CAD build for the part. Positions are in the model's coordinates, mm. Face numbers are marked on the shaded views. A direction names the side the tool comes from. Give positions to 0.01 mm unless a question says otherwise; leave off trailing zeros. Order: outer loops, then holes, each group sorted by start corner. A loop starts at its lowest first (then second) coordinate and runs counter-clockwise, first axis right, second up.
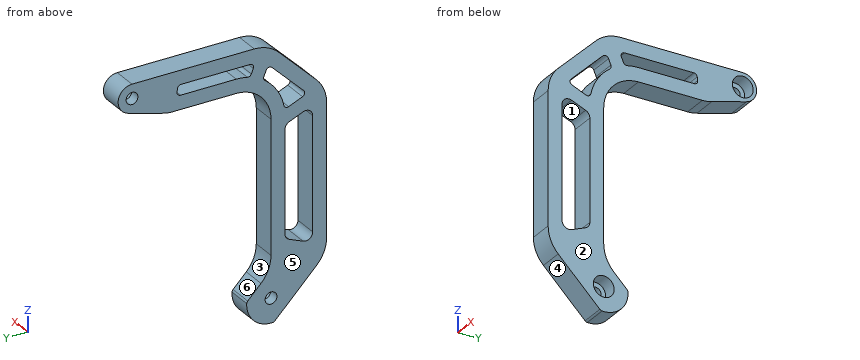
Autodesk Inventor part; units mm, degrees
ref_plane "YZ Plane" through (0, 0, 0) normal (1, 0, 0) x (0, 1, 0)
ref_plane "XZ Plane" through (0, 0, 0) normal (0, 1, 0) x (-1, 0, 0)
ref_plane "XY Plane" through (0, 0, 0) normal (0, 0, 1) x (1, 0, 0)
sketch "SwingArm A" plane through (0, 0, 0) normal (0, 0, 1) x (1, 0, 0)
  line L0 (-13.1129, 5.4447) -> (-1.1226, -6.6888)
  arc A0 (6.9887, 0.3969) -> (6.7016, 1.0431) centre (5.9903, 0.3402) ccw
  arc A1 (-1.1226, -6.6888) -> (-0.4798, -6.9835) centre (-0.4113, -5.9859) ccw
  line L1 (40, 71) -> (4.8211, 71)
  line L2 (28.3926, 60) -> (0, 60) construction
  line L3 (-2.2079, 68.1129) -> (-13.029, 57.4195)
  line L4 (-16, 50.3066) -> (-16, 12.4737)
  line L5 (0, 60) -> (0, 11.9322) construction
  line L6 (2.8871, 4.9032) -> (6.7016, 1.0431)
  circle A2 centre (0, 0) radius 1.7
  circle A3 centre (40, 67) radius 1.7
  line L7 (40, 67) -> (-8, 67) construction
  line L8 (-8, 67) -> (-8, 8.0955) construction
  line L9 (-8, 8.0955) -> (0, 0) construction
  line L10 (41.0716, 63.1462) -> (31.0716, 60.3655)
  arc A4 (28.3926, 60) -> (31.0716, 60.3655) centre (28.3926, 70) ccw
  circle A5 centre (40, 67) radius 4 construction
  arc A6 (41.0716, 63.1462) -> (40, 71) centre (40, 67) ccw
  circle A7 centre (0, 0) radius 5.5 construction
  arc A8 (10, 60) -> (0, 50) centre (10, 50) ccw
  arc A9 (0, 11.9322) -> (2.8871, 4.9032) centre (10, 11.9322) ccw
  arc A10 (-16, 12.4737) -> (-13.1129, 5.4447) centre (-6, 12.4737) ccw
  arc A11 (-13.029, 57.4195) -> (-16, 50.3066) centre (-6, 50.3066) ccw
  arc A12 (4.8211, 71) -> (-2.2079, 68.1129) centre (4.8211, 61) ccw
  line L11 (-9.2401, 13.305) -> (-5.2401, 14.948)
  line L12 (-4, 16.798) -> (-4, 45.9717)
  line L13 (-5.2292, 47.8172) -> (-9.2292, 49.488)
  line L14 (-12, 47.6425) -> (-12, 15.155)
  arc A13 (-4, 45.9717) -> (-5.2292, 47.8172) centre (-6, 45.9717) ccw
  arc A14 (-9.2292, 49.488) -> (-12, 47.6425) centre (-10, 47.6425) ccw
  arc A15 (-5.2401, 14.948) -> (-4, 16.798) centre (-6, 16.798) ccw
  arc A16 (-12, 15.155) -> (-9.2401, 13.305) centre (-10, 15.155) ccw
  line L15 (28.3926, 60) -> (10, 60)
  line L16 (0, 50) -> (0, 11.9322)
  line L17 (1.3855, 64.1003) -> (2.0531, 62.4749)
  line L18 (-5.0798, 52.0897) -> (-9.0729, 53.7576)
  line L19 (-0.2424, 64.4316) -> (-9.3904, 55.3916)
  arc A17 (1.7195, 61.2887) -> (2.0531, 62.4749) centre (1.1281, 62.095) ccw
  arc A18 (1.3855, 64.1003) -> (-0.2424, 64.4316) centre (0.4605, 63.7204) ccw
  arc A19 (-5.0798, 52.0897) -> (-3.7148, 52.8116) centre (-4.6944, 53.0125) ccw
  arc A20 (-9.3904, 55.3916) -> (-9.0729, 53.7576) centre (-8.6875, 54.6803) ccw
  line L20 (-15.2274, 54.1608) -> (0, 47.8005) construction
  arc A21 (-0.4798, -6.9835) -> (6.9887, 0.3969) centre (0, 0) ccw
  arc A22 (1.7195, 61.2887) -> (-3.7148, 52.8116) centre (10, 50) ccw
  line L21 (0.0419, 2.0916) -> (2.8931, -0.7936) construction
  arc A23 (0.7592, -2.9023) -> (2.8931, -0.7936) centre (0, 0) ccw construction
  line L22 (0.7592, -2.9023) -> (-10.2677, 8.2563) construction
  arc A24 (-12, 12.4737) -> (-10.2677, 8.2563) centre (-6, 12.4737) ccw construction
  line L23 (-12, 12.4737) -> (-12, 50.3066) construction
  arc A25 (-10.2174, 54.5744) -> (-12, 50.3066) centre (-6, 50.3066) ccw construction
  line L24 (-10.2174, 54.5744) -> (0.6037, 65.2677) construction
  arc A26 (4.8211, 67) -> (0.6037, 65.2677) centre (4.8211, 61) ccw construction
  line L25 (4.8211, 67) -> (40, 67) construction
  line L26 (40, 67) -> (30, 64.2193) construction
  arc A27 (28.3926, 64) -> (30, 64.2193) centre (28.3926, 70) ccw construction
  line L27 (28.3926, 64) -> (10, 64) construction
  arc A28 (10, 64) -> (-4, 50) centre (10, 50) ccw construction
  line L28 (-4, 50) -> (-4, 11.9322) construction
  arc A29 (-4, 11.9322) -> (0.0419, 2.0916) centre (10, 11.9322) ccw construction
  line L29 (-15.2501, 8.6743) -> (0, 14.9381) construction
  line L30 (1.0217, 70.2501) -> (5.6423, 59.0006) construction
  line L31 (29.7445, 60.0918) -> (28.2561, 71) construction
  line L32 (5.6582, 64.2257) -> (5.0855, 65.6201)
  line L33 (26.9014, 66.1352) -> (27.0378, 65.1352)
  line L34 (25.9106, 67) -> (6.0106, 67)
  line L35 (26.047, 64) -> (10, 64)
  arc A30 (10, 64) -> (6.811, 63.632) centre (10, 50) ccw
  arc A31 (5.6582, 64.2257) -> (6.811, 63.632) centre (6.5833, 64.6057) ccw
  arc A32 (6.0106, 67) -> (5.0855, 65.6201) centre (6.0106, 66) ccw
  arc A33 (26.9014, 66.1352) -> (25.9106, 67) centre (25.9106, 66) ccw
  arc A34 (26.047, 64) -> (27.0378, 65.1352) centre (26.047, 65) ccw
  point P0 (-12, 31.3902)
  point P1 (-16, 31.3902)
  dimension "d0" = 3.4
  dimension "d1" = 3.4
  dimension "d2" = 7
  dimension "d3" = 4
  dimension "d6" = 10
  dimension "d7" = 16
  dimension "d8" = 67
  dimension "d9" = 10
  dimension "d10" = 10
  dimension "d11" = 10
  dimension "d12" = 10
  dimension "d13" = 10
  dimension "d14" = 40
  dimension "d15" = 134.66
  dimension "d16" = 2
  dimension "d17" = 2
  dimension "d18" = 1
  dimension "d20" = 4
  dimension "d24" = 10
  dimension "d25" = 50
  dimension "d32" = 7
  dimension "d33" = 11
  dimension "d34" = 1
  dimension "d35" = 4
  dimension "d37" = 2
  dimension "d38" = 4
  dimension "d39" = 1
  dimension "d41" = 2
  dimension "d42" = 1
  dimension "d43" = 1
sketch "Skizze1" plane through (0, 0, 0) normal (1, 0, 0) x (0, 1, 0)
  circle A0 centre (40, 67) radius 3
  circle A1 centre (0, 0) radius 3
  line L0 (-13.1129, 5.4447) -> (-1.1226, -6.6888)
  arc A2 (6.9887, 0.3969) -> (6.7016, 1.0431) centre (5.9903, 0.3402) ccw
  arc A3 (-1.1226, -6.6888) -> (-0.4798, -6.9835) centre (-0.4113, -5.9859) ccw
  line L1 (40, 71) -> (4.8211, 71)
  line L2 (28.3926, 60) -> (0, 60) construction
  line L3 (-2.2079, 68.1129) -> (-13.029, 57.4195)
  line L4 (-16, 50.3066) -> (-16, 12.4737)
  line L5 (0, 60) -> (0, 11.9322) construction
  line L6 (2.8871, 4.9032) -> (6.7016, 1.0431)
  circle A4 centre (0, 0) radius 1.7
  circle A5 centre (40, 67) radius 1.7
  line L7 (40, 67) -> (-8, 67) construction
  line L8 (-8, 67) -> (-8, 8.0955) construction
  line L9 (-8, 8.0955) -> (0, 0) construction
  line L10 (41.0716, 63.1462) -> (31.0716, 60.3655)
  arc A6 (28.3926, 60) -> (31.0716, 60.3655) centre (28.3926, 70) ccw
  circle A7 centre (40, 67) radius 4 construction
  arc A8 (41.0716, 63.1462) -> (40, 71) centre (40, 67) ccw
  circle A9 centre (0, 0) radius 5.5 construction
  arc A10 (10, 60) -> (0, 50) centre (10, 50) ccw
  arc A11 (0, 11.9322) -> (2.8871, 4.9032) centre (10, 11.9322) ccw
  arc A12 (-16, 12.4737) -> (-13.1129, 5.4447) centre (-6, 12.4737) ccw
  arc A13 (-13.029, 57.4195) -> (-16, 50.3066) centre (-6, 50.3066) ccw
  arc A14 (4.8211, 71) -> (-2.2079, 68.1129) centre (4.8211, 61) ccw
  line L11 (-9.2401, 13.305) -> (-5.2401, 14.948)
  line L12 (-4, 16.798) -> (-4, 45.9717)
  line L13 (-5.2292, 47.8172) -> (-9.2292, 49.488)
  line L14 (-12, 47.6425) -> (-12, 15.155)
  arc A15 (-4, 45.9717) -> (-5.2292, 47.8172) centre (-6, 45.9717) ccw
  arc A16 (-9.2292, 49.488) -> (-12, 47.6425) centre (-10, 47.6425) ccw
  arc A17 (-5.2401, 14.948) -> (-4, 16.798) centre (-6, 16.798) ccw
  arc A18 (-12, 15.155) -> (-9.2401, 13.305) centre (-10, 15.155) ccw
  line L15 (28.3926, 60) -> (10, 60)
  line L16 (0, 50) -> (0, 11.9322)
  line L17 (1.3855, 64.1003) -> (2.0531, 62.4749)
  line L18 (-5.0798, 52.0897) -> (-9.0729, 53.7576)
  line L19 (-0.2424, 64.4316) -> (-9.3904, 55.3916)
  arc A19 (1.7195, 61.2887) -> (2.0531, 62.4749) centre (1.1281, 62.095) ccw
  arc A20 (1.3855, 64.1003) -> (-0.2424, 64.4316) centre (0.4605, 63.7204) ccw
  arc A21 (-5.0798, 52.0897) -> (-3.7148, 52.8116) centre (-4.6944, 53.0125) ccw
  arc A22 (-9.3904, 55.3916) -> (-9.0729, 53.7576) centre (-8.6875, 54.6803) ccw
  line L20 (-15.2274, 54.1608) -> (0, 47.8005) construction
  arc A23 (-0.4798, -6.9835) -> (6.9887, 0.3969) centre (0, 0) ccw
  arc A24 (1.7195, 61.2887) -> (-3.7148, 52.8116) centre (10, 50) ccw
  line L21 (0.0419, 2.0916) -> (2.8931, -0.7936) construction
  arc A25 (0.7592, -2.9023) -> (2.8931, -0.7936) centre (0, 0) ccw construction
  line L22 (0.7592, -2.9023) -> (-10.2677, 8.2563) construction
  arc A26 (-12, 12.4737) -> (-10.2677, 8.2563) centre (-6, 12.4737) ccw construction
  line L23 (-12, 12.4737) -> (-12, 50.3066) construction
  arc A27 (-10.2174, 54.5744) -> (-12, 50.3066) centre (-6, 50.3066) ccw construction
  line L24 (-10.2174, 54.5744) -> (0.6037, 65.2677) construction
  arc A28 (4.8211, 67) -> (0.6037, 65.2677) centre (4.8211, 61) ccw construction
  line L25 (4.8211, 67) -> (40, 67) construction
  line L26 (40, 67) -> (30, 64.2193) construction
  arc A29 (28.3926, 64) -> (30, 64.2193) centre (28.3926, 70) ccw construction
  line L27 (28.3926, 64) -> (10, 64) construction
  arc A30 (10, 64) -> (-4, 50) centre (10, 50) ccw construction
  line L28 (-4, 50) -> (-4, 11.9322) construction
  arc A31 (-4, 11.9322) -> (0.0419, 2.0916) centre (10, 11.9322) ccw construction
  line L29 (-15.2501, 8.6743) -> (0, 14.9381) construction
  line L30 (1.0217, 70.2501) -> (5.6423, 59.0006) construction
  line L31 (29.7445, 60.0918) -> (28.2561, 71) construction
  line L32 (5.6582, 64.2257) -> (5.0855, 65.6201)
  line L33 (26.9014, 66.1352) -> (27.0378, 65.1352)
  line L34 (25.9106, 67) -> (6.0106, 67)
  line L35 (26.047, 64) -> (10, 64)
  arc A32 (10, 64) -> (6.811, 63.632) centre (10, 50) ccw
  arc A33 (5.6582, 64.2257) -> (6.811, 63.632) centre (6.5833, 64.6057) ccw
  arc A34 (6.0106, 67) -> (5.0855, 65.6201) centre (6.0106, 66) ccw
  arc A35 (26.9014, 66.1352) -> (25.9106, 67) centre (25.9106, 66) ccw
  arc A36 (26.047, 64) -> (27.0378, 65.1352) centre (26.047, 65) ccw
  dimension "d44" = 6
  dimension "d45" = 6
extrude "Extrusion1" add sketch "Skizze1" along normal blind 4 and the other way blind 3 contours A0 | A1 | A12 L4 A13 L3 A14 L1 A8 L10 A6 L15 A10 L16 A11 L6 A2 A23 A3 L0
extrude "Extrusion2" cut sketch "Skizze1" along normal through all contours A0 | A1
properties part number "Swing-Arm A" material "ABS-Kunststoff"
1. Saw through at B-B on x = 3. State how many separate pieces and enclosed holes the cut face has, plus the area to 3 significant figures.
2. Saw through at C-C on z = 8.5. Give the cut face in (x, y), plus the area to 3 significant figures.
3. Wall check: line 1 (Z direction, x = -0.25, y = 10); line 2 (Z direction, x = 3.75, y = -1.5); line 3 (Z direction, x = 3.25, y = -7.5). Give the ranges that are in metal, low to high.
4. Saw through at A-A on z = 20. Give the cut face in (x, y).
5. 3-axis set-ups, long thin cutter, end or side, ignore diameter. For the marked faces 1, 2 and 3: which of +Z, -Z, +X, -X, +Y, -Y reach the whole face in a straight line?
6. Pin check, flat tips, straight feed: P1, Ø2, axis at x = -2, z = 21, coming from the +Y side; P2, Ø1.8, axis at y = 40.5, z = 65.5, coming from the +X side. Stop position of each tip, or through.
7. Mould opens along Z. For the marked faces 4, 5 and 6 say: released by +Z, released by -Z, zero draft, split by the parting line, or undercut.
Reported:
1. separate pieces: 1
1. enclosed holes: 5
1. area: 1,070 mm2
2. outline: (-3, -15.18) - (4, -15.18) - (4, 0.61) - (-3, 0.61) - close
2. area: 110 mm2
3. line 1: z = 60 to 64, 67 to 71
3. line 2: z = -6.31 to -2.6, 2.6 to 57.98, 63.19 to 68.75
3. line 3: z = -0.24 to 14.02, 48.77 to 53.1, 57.26 to 62.88
4. outline: (-3, -16) - (4, -16) - (4, -12) - (-3, -12) - close; (-3, -4) - (4, -4) - (4, 0) - (-3, 0) - close
5. face 1: +X, -X
5. face 2: +Z, -Z, +X, +Y, -Y
5. face 3: +X, -X, +Y
6. P1: stops at y = 0
6. P2: stops at x = 0
7. face 4: released by -Z
7. face 5: zero draft
7. face 6: undercut
